Could you check a few things on this model? Use its own coordinates, in mm. A direction names the side the tool comes from. Coordinates: 2 decimals unless noted, no trailing zeros. Write each loop counter-clockwise with the first axis right and the second up, starting at its lowest first coordinate (ties: lowest second). Pieces come first, ordered by that corner, then holes. Notation, with made-up numbers: M 69,26 L 116,26 A17 cw 116,35 Z; hole C 56.25,-12 d5. An arc over 180 degrees is marked long. Answer as CSV lines item,"result". Start each with the question number.
Item 1: We'd pull the mould along X, two halves only. Please class faces 3 (the cylindrical face through (0.62, 5.07, -24.02)), 4 (the flat face through (-12.5, 5, 1)), 5 (the cylindrical face through (11.297, 5.07, 48.859)): +X half, -X half, draft (parallel to the pull), parting line (faces both ways), or undercut.
Item 2: Suppose I cut it at C-C, the plane z = 27. Write out the boundary of the cut face in (x, y) (3 decimals).
Item 3: Suppose I cut it at D-D, the plane x = -11. Write out the boundary of the cut face in (y, z).
Item 4: Suppose I cut it at A-A, the plane z = -34. Write out the boundary of the cut face in (x, y) (3 decimals), and give its area (4 significant figures).
Item 5: Suppose I cut it at B-B, the plane y = 4. State how many separate pieces and enclosed holes the cut face has, and give its area (3 significant figures).
Item 6: If I drill on line 1 along Z through (x, y) = (1, 8); line 2 along X through (y, z) = (5, -34) (3 decimals); line 3 along Z through (x, y) = (1.5, 1), over which ranges is the centre line in solid material (lowest first)? Write a range as [from, to].
Item 7: I'm going to push a flat-ended pin straight in: P1, Ø6.5, axis at x = 0, z = -42, coming from the +Y side. Where does the tip first touch, or does it pass through?
Item 8: On a 3-axis mill with a long thin cutter (end or side, diameter ignored), from which of +Z, -Z, +X, -X, +Y, -Y can I reach the whole of each face in a straight line? I mean faces 1 (the cylindrical face through (2.198, 5.07, -17.075)), 2 (the flat face through (0, 5, -50)). Say none if no direction works.
```python
from build123d import *

# Parameters (mm, degrees)
SKETCH1_W                    = 25
SKETCH1_H                    = 100
BOSS_EXTRUDE1_DEPTH          = 10
CUT_EXTRUDE_THIN2_DEPTH      = 53.5
CUT_EXTRUDE_THIN2_DEPTH_BACK = 10
SKETCH3_W                    = 6.15
SKETCH3_H                    = 60
FILLET2_R                    = 3.075
FILLET3_R                    = 4
SKETCH4_R                    = 2.075
CUT_EXTRUDE1_DEPTH           = 53.5
LPATTERN1_COUNT              = 3
LPATTERN1_PITCH              = 8


with BuildPart() as part:
    # Sketch1 → Boss-Extrude1 (new body)
    with BuildSketch(Plane(origin=(0, 0, 0), x_dir=(1, 0, 0), z_dir=(0, 1, 0))):
        Rectangle(SKETCH1_W, SKETCH1_H)
    extrude(amount=BOSS_EXTRUDE1_DEPTH)

    # Sketch3 → Cut-Extrude-Thin2 (cut, two sides: drawn at the far end of the back side and taken through both)
    with BuildSketch(Plane(origin=(0, 10, 0), x_dir=(1, 0, 0), z_dir=(0, 1, 0)).offset(-CUT_EXTRUDE_THIN2_DEPTH_BACK)):
        with Locations((0, -12)):
            Rectangle(SKETCH3_W, SKETCH3_H)
    extrude(amount=CUT_EXTRUDE_THIN2_DEPTH + CUT_EXTRUDE_THIN2_DEPTH_BACK, mode=Mode.SUBTRACT)

    # Fillet2
    fillet2_edges = [part.edges().sort_by_distance(p)[0] for p in [
        (3.075, 5, -18),
        (-3.075, 5, -18),
        (3.075, 5, 42),
        (-3.075, 5, 42),
    ]]
    fillet(fillet2_edges, radius=FILLET2_R - 0.0001)  # a hair under: the kernel refuses the full size

    # Fillet3
    fillet3_edges = [part.edges().sort_by_distance(p)[0] for p in [
        (12.5, 5, 50),
        (-12.5, 5, 50),
        (-12.5, 5, -50),
        (12.5, 5, -50),
    ]]
    fillet(fillet3_edges, radius=FILLET3_R)

    # Sketch4 → Cut-Extrude1 (cut, through all)
    with BuildSketch(Plane(origin=(0, 10, 0), x_dir=(1, 0, 0), z_dir=(0, 1, 0))):
        with Locations(Location((0, 42, 0), (0, 0, 270))):
            Circle(SKETCH4_R)
    cut_extrude1 = extrude(amount=-CUT_EXTRUDE1_DEPTH, mode=Mode.SUBTRACT)

    # LPattern1: Cut-Extrude1 ×3
    with Locations(*[(0, 0, i * LPATTERN1_PITCH) for i in range(1, LPATTERN1_COUNT)]):
        add(cut_extrude1, mode=Mode.SUBTRACT)


solid = part.part
```
Ans:
1,face 3,"undercut"
1,face 4,"-X half"
1,face 5,"+X half"
2,outline,"M -12.5,0 L -3.075,0 L -3.075,10 L -12.5,10 Z; M 3.075,0 L 12.5,0 L 12.5,10 L 3.075,10 Z"
3,outline,"M 0,-49.12 L 10,-49.12 L 10,49.12 L 0,49.12 Z"
4,outline,"M -12.5,0 L -2.075,0 L -2.075,10 L -12.5,10 Z; M 2.075,0 L 12.5,0 L 12.5,10 L 2.075,10 Z"
4,area,"208.5 mm^2"
5,separate pieces,"1"
5,enclosed holes,"4"
5,area,"2,080 mm^2"
6,line 1,"z = [-50, -43.82], [-40.18, -35.82], [-32.18, -27.82], [-24.18, -17.83], [41.83, 50]"
6,line 2,"x = [-12.5, -2.075], [2.075, 12.5]"
6,line 3,"z = [-50, -43.43], [-40.57, -35.43], [-32.57, -27.43], [-24.57, -17.61], [41.61, 50]"
7,P1,"stops at y = 10"
8,face 1,"+Y, -Y"
8,face 2,"-Z, +X, -X, +Y, -Y"
